Can you work these out from the drawing? Everything is in mm from the part's minimum corner. A direction names the side the tool comes from. Give positions to 0.01 mm unless a question says otherwise; leave off trailing zeros. Loops run counter-clockwise (first coordinate to the right, second up) from the corner with the lowest first, then second, coordinate; pieces in that order, holes last. Notation, with made-up numbers: (64, 20.25) - (87, 20.25) arc R22 cw to (87, 28.25) - close; hole circle Ø2 at (59, 85.5). An arc over 180 degrees is marked (long way). One line per item, written item: value. Start each with the question number.
Q1. If we mould it in two halves opening along Y, with no side actions, what happens to the marked faces 1, 2 and 3? For each: released by +Y, released by -Y, zero draft, split by the parting line, or undercut.
Q2. I want a section at A-A (z = 4.5). Please give me the cut outline in (x, y), then the cut area to 3 significant figures.
Q3. If I drill on line 1 (X direction, y = 39, z = 18); line 2 (Z direction, x = 56, y = 38); line 3 (X direction, y = 6, z = 25), over which ranges is the centre line in solid material (lowest first)? Write a range as from..to.
Q4. I'm going to push flat-ended pins straight in: P1, Ø2, axis at x = 27, z = 18, coming from the +Y side; P2, Ø11, axis at x = 3.5, z = 15, coming from the +Y side; P3, Ø3, axis at x = 44, z = 25, coming from the +Y side. Where does each tip first touch, or does it pass through?
Q5. I want a section at C-C (x = 44). Please give me the cut outline in (y, z).
Q6. I want a section at B-B (x = 56). Please give me the cut outline in (y, z).
Q7. I want a section at D-D (z = 18). Please give me the cut outline in (x, y).
Q8. For the marked faces 4, 5 and 6, which set-ups out of +Z, -Z, +X, -X, +Y, -Y let a thin tool reach every point of the face, with its end or its side?
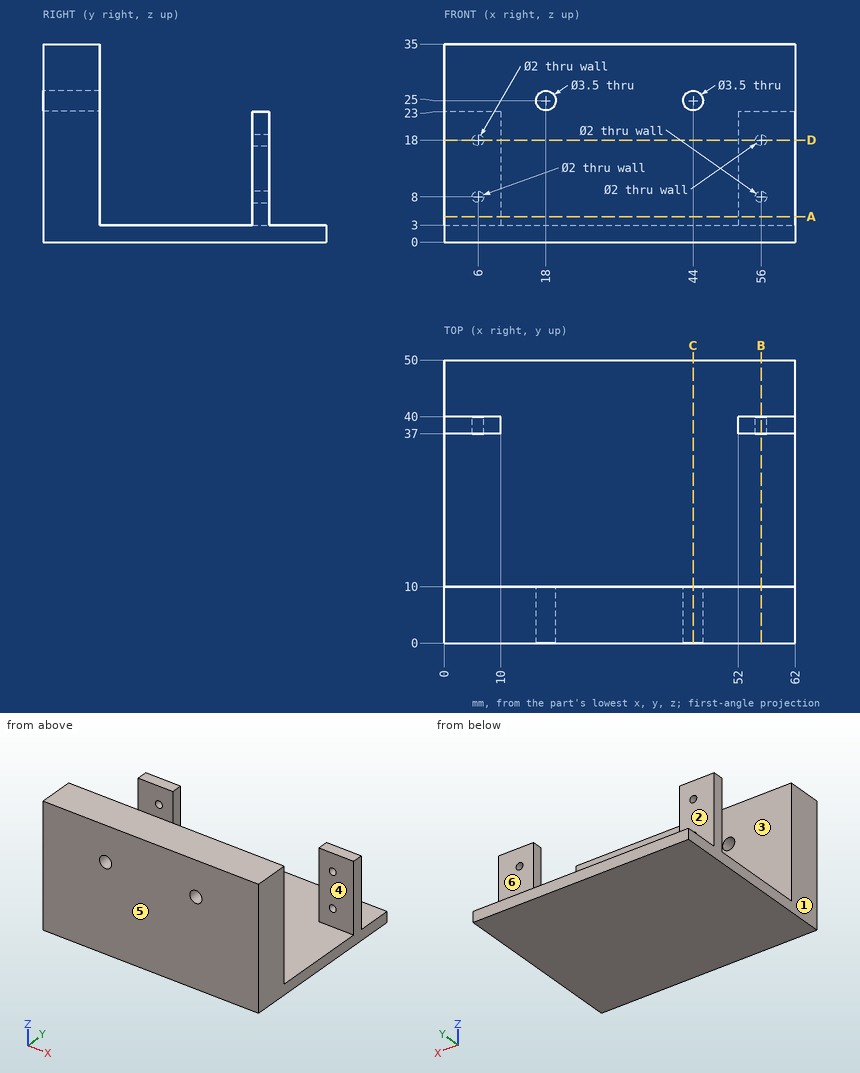
Worked answers:
1. face 1: zero draft
1. face 2: released by +Y
1. face 3: undercut
2. outline: (0, 0) - (62, 0) - (62, 10) - (0, 10) - close; (0, 37) - (10, 37) - (10, 40) - (0, 40) - close; (52, 37) - (62, 37) - (62, 40) - (52, 40) - close
2. area: 680 mm²
3. line 1: x = 0..5, 7..10, 52..55, 57..62
3. line 2: z = 0..7, 9..17, 19..23
3. line 3: x = 0..16.25, 19.75..42.25, 45.75..62
4. P1: stops at y = 10
4. P2: stops at y = 40
4. P3: passes through
5. outline: (0, 0) - (50, 0) - (50, 3) - (10, 3) - (10, 23.25) - (0, 23.25) - close; (0, 26.75) - (10, 26.75) - (10, 35) - (0, 35) - close
6. outline: (0, 0) - (50, 0) - (50, 3) - (40, 3) - (40, 7) - (37, 7) - (37, 3) - (10, 3) - (10, 35) - (0, 35) - close; (37, 9) - (40, 9) - (40, 17) - (37, 17) - close; (37, 19) - (40, 19) - (40, 23) - (37, 23) - close
7. outline: (0, 0) - (62, 0) - (62, 10) - (0, 10) - close; (0, 37) - (5, 37) - (5, 40) - (0, 40) - close; (7, 37) - (10, 37) - (10, 40) - (7, 40) - close; (52, 37) - (55, 37) - (55, 40) - (52, 40) - close; (57, 37) - (62, 37) - (62, 40) - (57, 40) - close
8. face 4: +Z, +X, -X
8. face 5: +Z, -Z, +X, -X, -Y
8. face 6: +Z, +X, -X, +Y
